from build123d import *

# Parameters (mm, degrees)
SKETCH2_R           = 4.137132353
BOSS_EXTRUDE1_DEPTH = 40
SKETCH2_4_R         = 22.521813525
BOSS_EXTRUDE2_DEPTH = 5
BOSS_EXTRUDE3_DEPTH = 35
SKETCH6_R           = 3.1
CUT_EXTRUDE1_DEPTH  = 17


with BuildPart() as part:
    # Sketch2 → Boss-Extrude1 (new body)
    with BuildSketch(Plane.XY.offset(-16.453858319)):
        Circle(SKETCH2_R)
    extrude(amount=BOSS_EXTRUDE1_DEPTH)

    # Sketch2<4> → Boss-Extrude2 (add)
    with BuildSketch(Plane.XY.offset(-16.453858319)):
        Circle(SKETCH2_4_R)
    extrude(amount=BOSS_EXTRUDE2_DEPTH)

    # Sketch5 → Boss-Extrude3 (add)
    with BuildSketch(Plane.XY.offset(-11.453858319)):
        with BuildLine():
            Line((3.09152076, 5.413957434), (2.594362934, 3.858987039))
            ThreePointArc((2.594362934, 3.858987039), (3.287908356, 3.288184703), (3.85876898, 2.594687257))
            Line((3.85876898, 2.594687257), (5.413697585, 3.091975771))
            ThreePointArc((5.413697585, 3.091975771), (5.765755257, 3.074104639), (6.018526007, 2.828399672))
            ThreePointArc((6.018526007, 2.828399672), (6.143691944, 2.545103004), (6.25553153, 2.256285725))
            ThreePointArc((6.25553153, 2.256285725), (6.250564892, 1.903809747), (6.014281308, 1.642210721))
            Line((6.014281308, 1.642210721), (4.563207527, 0.894224281))
            ThreePointArc((4.563207527, 0.894224281), (4.649999996, 0.000195407), (4.563282667, -0.893840758))
            Line((4.563282667, -0.893840758), (6.014419308, -1.641705239))
            ThreePointArc((6.014419308, -1.641705239), (6.250724877, -1.903284405), (6.25572114, -2.255759964))
            ThreePointArc((6.25572114, -2.255759964), (6.143905828, -2.544586642), (6.018763701, -2.827893829))
            ThreePointArc((6.018763701, -2.827893829), (5.766013604, -3.073620039), (5.413957434, -3.09152076))
            Line((5.413957434, -3.09152076), (3.858987039, -2.594362934))
            ThreePointArc((3.858987039, -2.594362934), (3.288184703, -3.287908356), (2.594687257, -3.85876898))
            Line((2.594687257, -3.85876898), (3.091975771, -5.413697585))
            ThreePointArc((3.091975771, -5.413697585), (3.074104639, -5.765755257), (2.828399672, -6.018526007))
            ThreePointArc((2.828399672, -6.018526007), (2.545103004, -6.143691944), (2.256285725, -6.25553153))
            ThreePointArc((2.256285725, -6.25553153), (1.903809747, -6.250564892), (1.642210721, -6.014281308))
            Line((1.642210721, -6.014281308), (0.894224281, -4.563207527))
            ThreePointArc((0.894224281, -4.563207527), (0.000195407, -4.649999996), (-0.893840758, -4.563282667))
            Line((-0.893840758, -4.563282667), (-1.641705239, -6.014419308))
            ThreePointArc((-1.641705239, -6.014419308), (-1.903284405, -6.250724877), (-2.255759964, -6.25572114))
            ThreePointArc((-2.255759964, -6.25572114), (-2.544586642, -6.143905828), (-2.827893829, -6.018763701))
            ThreePointArc((-2.827893829, -6.018763701), (-3.073620039, -5.766013604), (-3.09152076, -5.413957434))
            Line((-3.09152076, -5.413957434), (-2.594362934, -3.858987039))
            ThreePointArc((-2.594362934, -3.858987039), (-3.287908356, -3.288184703), (-3.85876898, -2.594687257))
            Line((-3.85876898, -2.594687257), (-5.413697585, -3.091975771))
            ThreePointArc((-5.413697585, -3.091975771), (-5.765755257, -3.074104639), (-6.018526007, -2.828399672))
            ThreePointArc((-6.018526007, -2.828399672), (-6.143691944, -2.545103004), (-6.25553153, -2.256285725))
            ThreePointArc((-6.25553153, -2.256285725), (-6.250564892, -1.903809747), (-6.014281308, -1.642210721))
            Line((-6.014281308, -1.642210721), (-4.563207527, -0.894224281))
            ThreePointArc((-4.563207527, -0.894224281), (-4.649999996, -0.000195407), (-4.563282667, 0.893840758))
            Line((-4.563282667, 0.893840758), (-6.014419308, 1.641705239))
            ThreePointArc((-6.014419308, 1.641705239), (-6.250724877, 1.903284405), (-6.25572114, 2.255759964))
            ThreePointArc((-6.25572114, 2.255759964), (-6.143905828, 2.544586642), (-6.018763701, 2.827893829))
            ThreePointArc((-6.018763701, 2.827893829), (-5.766013604, 3.073620039), (-5.413957434, 3.09152076))
            Line((-5.413957434, 3.09152076), (-3.858987039, 2.594362934))
            ThreePointArc((-3.858987039, 2.594362934), (-3.288184703, 3.287908356), (-2.594687257, 3.85876898))
            Line((-2.594687257, 3.85876898), (-3.091975771, 5.413697585))
            ThreePointArc((-3.091975771, 5.413697585), (-3.074104639, 5.765755257), (-2.828399672, 6.018526007))
            ThreePointArc((-2.828399672, 6.018526007), (-2.545103004, 6.143691944), (-2.256285725, 6.25553153))
            ThreePointArc((-2.256285725, 6.25553153), (-1.903809747, 6.250564892), (-1.642210721, 6.014281308))
            Line((-1.642210721, 6.014281308), (-0.894224281, 4.563207527))
            ThreePointArc((-0.894224281, 4.563207527), (-0.000195407, 4.649999996), (0.893840758, 4.563282667))
            Line((0.893840758, 4.563282667), (1.641705239, 6.014419308))
            ThreePointArc((1.641705239, 6.014419308), (1.903284405, 6.250724877), (2.255759964, 6.25572114))
            ThreePointArc((2.255759964, 6.25572114), (2.544586642, 6.143905828), (2.827893829, 6.018763701))
            ThreePointArc((2.827893829, 6.018763701), (3.073620039, 5.766013604), (3.09152076, 5.413957434))
        make_face()
    extrude(amount=BOSS_EXTRUDE3_DEPTH)

    # Sketch6 → Cut-Extrude1 (cut)
    with BuildSketch(Plane(origin=(0, 0, -16.453858319), x_dir=(-1, 0, 0), z_dir=(0, 0, -1))):
        Circle(SKETCH6_R)
    extrude(amount=-CUT_EXTRUDE1_DEPTH, mode=Mode.SUBTRACT)


solid = part.part
The listing builds one solid part. Answer for the finished solid, in the listing's coordinates (mm). A direction names the side the tool comes from. Coordinates: 2 decimals unless noted, no trailing zeros. Loops run counter-clockwise (first coordinate to the right, second up) from the corner with the lowest first, then second, coordinate; pieces in that order, holes last.
1) Find section D-D on y = -17.5. Write down the section's boundary in (x, z), then the cut area to 3 significant figures.
2) Flat-ended cylindrical pins translate along their axes: pin 1 Ø3 at (x, y) = (0, 0.5) entering from -Z; pin 2 Ø7 at (x, y) = (0, 0) entering from -Z; pin 3 Ø4 at (x, y) = (11.5, 13) entering from +Z; pin 4 Ø12 at (x, z) = (0.5, 3.5) entering from -Y. Find the tip coordinate at first contact, or state that the pin passes through.
3) Find section C-C on x = -14. Write down the section's boundary in (y, z).
4) Find section A-A on y = 0. Write down the section's boundary in (x, z).
5) Determine the mould class of faces 6 (the face through (4.63, 2.84, 5.8)), 7 (the face through (-3.279, -3.297, 5.801)), 8 (the face through (5, 0, -16.454)), 9 (the face through (-4.63, -2.84, 5.8)) for opening direction Y: pulls with the +Y half, pulls with the -Y half, needs draft (parallel to the pull), parting line crosses it, or undercut.
6) Find the intervals of material crossed by L1, parallel to Y at x = 0, z = -9; L2, parallel to Z at x = 9, y = -17; L3, parallel to Y at x = 0, z = -12, in increasing order.
7) A tool of negligible diameter and unlimited length cuts with its end or side. For faces 1 (the face through (-3.297, 3.279, 5.801)), 2 (the face through (-1.43, -2.75, -8.07)), 3 (the face through (0.01, -4.65, 5.8)), 4 (the face through (4.65, 0.01, 5.8)), 5 (the face through (-0.01, 4.65, 5.8)), from which of +Z, -Z, +X, -X, +Y, -Y can it reach the whole face along a straight path? Write none if from no direction.
Values:
1. outline: (-14.18, -16.45) - (14.18, -16.45) - (14.18, -11.45) - (-14.18, -11.45) - close
1. area: 142 mm2
2. pin 1: stops at z = 0.55
2. pin 2: stops at z = -16.45
2. pin 3: stops at z = -11.45
2. pin 4: stops at y = -6.29
3. outline: (-17.64, -16.45) - (17.64, -16.45) - (17.64, -11.45) - (-17.64, -11.45) - close
4. outline: (-22.52, -16.45) - (-3.1, -16.45) - (-3.1, 0.55) - (3.1, 0.55) - (3.1, -16.45) - (22.52, -16.45) - (22.52, -11.45) - (4.65, -11.45) - (4.65, 23.55) - (-4.65, 23.55) - (-4.65, -11.45) - (-22.52, -11.45) - close
5. face 6: pulls with the +Y half
5. face 7: undercut
5. face 8: needs draft
5. face 9: pulls with the -Y half
6. L1: y = -4.65 to -3.1, 3.1 to 4.65
6. L2: z = -16.45 to -11.45
6. L3: y = -22.52 to -3.1, 3.1 to 22.52
7. face 1: +Z
7. face 2: -Z
7. face 3: +Z, -Y
7. face 4: +Z, +X
7. face 5: +Z, +Y
